Design review of the part shown in the three views and the two pictorial views. Dimensions are in mm from the part's minimum x, y and z. Round coordinates to 2 decimals unless told otherwise and drop trailing zeros. Loops run counter-clockwise (first coordinate to the right, second up) from the corner with the lowest first, then second, coordinate; pieces in that order, holes last.
1. To check wall thickness, follow line 1 along Z through (x, y) = (6.5, 12.25); line 2 along X through (y, z) = (7, 6.5); line 3 along Y through (x, z) = (10.25, 2.75). State the ranges of each line that lie inside material, in increasing order.
2. Consider section C-C on y = 13. State the section outline as (x, z) points, then the cut area to 3 significant figures.
3. Consider section D-D on z = 1.75. State the section outline as (x, y) points, then the cut area to 3 significant figures.
4. Clearance check with flat-ended pins moving along their axes: pin 1 Ø1.5 at (x, y) = (10, 15.5) entering from +Z; pin 2 Ø6 at (y, z) = (3, 3) entering from +X; pin 3 Ø5 at (x, z) = (2.5, 6) entering from +Y; pin 4 Ø3 at (y, z) = (13.5, 9.5) entering from +X. State where each tip first meets the part, or that it passes through.
5. Consider section A-A on x = 6.5. State the section outline as (y, z) points.
6. Draft analysis for pull direction Z (two halves, no side actions). For the marked faces 1, 2 and 3, state which applies: released by +Z, released by -Z, zero draft, split by the parting line, or undercut.
7. Consider section B-B on z = 6.5. State the section outline as (x, y) points.
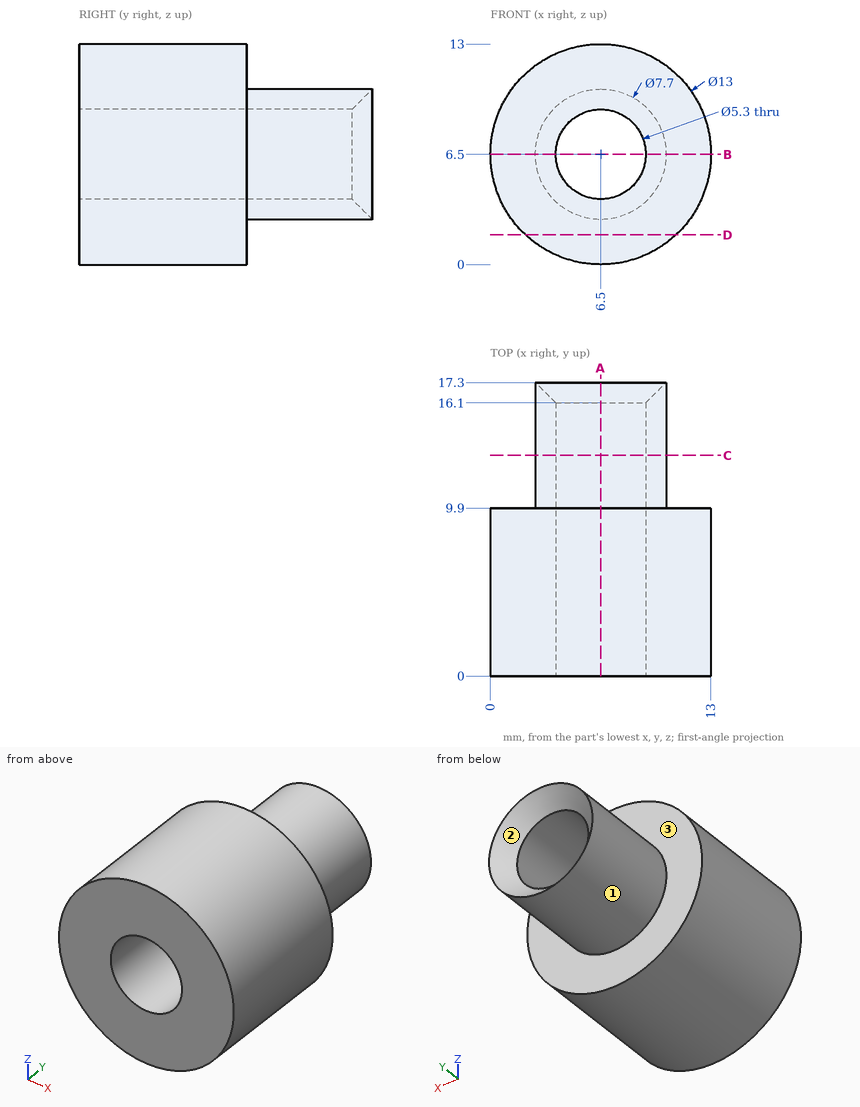
Resolved:
1. line 1: z = 2.65 to 3.85, 9.15 to 10.35
1. line 2: x = 0 to 3.85, 9.15 to 13
1. line 3: y = 0 to 9.9
2. outline: circle Ø7.7 at (6.5, 6.5); hole circle Ø5.3 at (6.5, 6.5)
2. area: 24.5 mm2
3. outline: (2.06, 0) - (10.94, 0) - (10.94, 9.9) - (2.06, 9.9) - close
3. area: 87.9 mm2
4. pin 1: stops at z = 9.19
4. pin 2: stops at x = 12.98
4. pin 3: stops at y = 17.3
4. pin 4: stops at x = 10.05
5. outline: (0, 0) - (9.9, 0) - (9.9, 2.65) - (17.3, 2.65) - (16.1, 3.85) - (0, 3.85) - close; (0, 9.15) - (16.1, 9.15) - (17.3, 10.35) - (9.9, 10.35) - (9.9, 13) - (0, 13) - close
6. face 1: split by the parting line
6. face 2: undercut
6. face 3: zero draft
7. outline: (0, 0) - (3.85, 0) - (3.85, 16.1) - (2.65, 17.3) - (2.65, 9.9) - (0, 9.9) - close; (9.15, 0) - (13, 0) - (13, 9.9) - (10.35, 9.9) - (10.35, 17.3) - (9.15, 16.1) - close
